The drawing under review shows one solid part. Ordinate dimensions are in mm from its lowest x, y, z. A direction names the side the tool comes from. Round coordinates to 2 decimals unless told otherwise and drop trailing zeros. Order: outer loops, then holes, each group sorted by start corner. A loop starts at its lowest first (then second) coordinate and runs counter-clockwise, first axis right, second up.
1) Clearance check with flat-ended pins moving along their axes: P1, Ø6.5, axis at x = 9, y = 139, coming from the -Z side (1 decimal); P2, Ø6.5, axis at x = 6.5, y = 133.5, coming from the +Z side; P3, Ø1.5, axis at x = 7.5, y = 106.5, coming from the +Z side. State where each tip first meets the part, or that it passes through.
2) To check wall thickness, follow L1, parallel to Y at x = 5, z = 19.5 (1 decimal); L2, parallel to Y at x = 1.5, z = 8 (1 decimal); L3, parallel to Z at x = 7.5, y = 35.5 (1 decimal). State the ranges of each line that lie inside material, in increasing order.
3) Machinability: for the marked faces 1, 2 and 3, which of the approach directions +Z, -Z, +X, -X, +Y, -Y give a long, thin tool a straight path to every point of the face, cutting with its end or side? Answer none if there is none.
4) Consider section C-C (z = 24). Give the boundary of the cut face in (x, y), then the cut area to 3 significant figures.
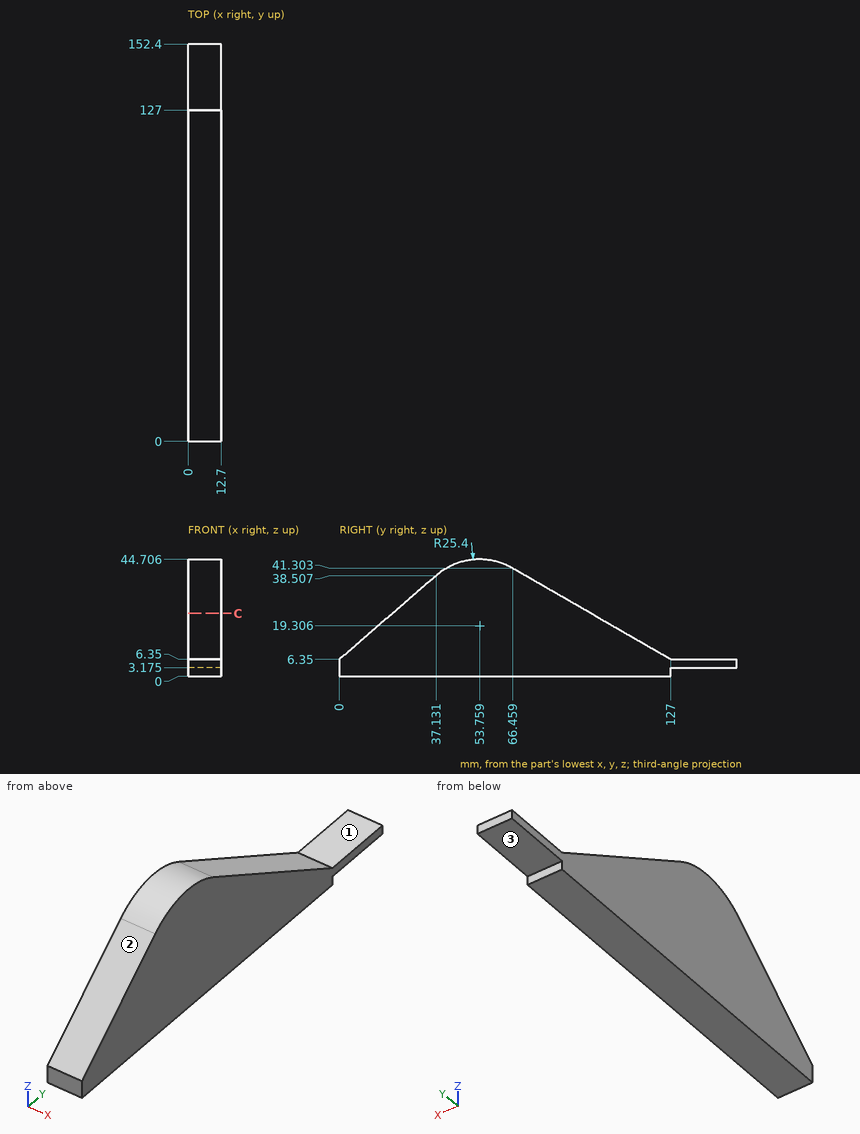
Answer below:
1. P1: stops at z = 3.2
1. P2: stops at z = 6.35
1. P3: stops at z = 18.62
2. L1: y = 15.2 to 104.2
2. L2: y = 1.9 to 124.1
2. L3: z = 0 to 37.1
3. face 1: +Z, +X, -X, +Y
3. face 2: +Z, +X, -X, -Y
3. face 3: -Z, +X, -X, +Y
4. outline: (0, 20.38) - (12.7, 20.38) - (12.7, 96.43) - (0, 96.43) - close
4. area: 966 mm2
